```python
from build123d import *

# Parameters (mm, degrees)
ESQUISSE1_R             = 1.5
ESQUISSE1_R_2           = 0.975
BOSS_EXTRU_3_DEPTH      = 2
ESQUISSE2_R             = 1.5
ENL_V_MAT_EXTRU_1_DEPTH = 10


with BuildPart() as part:
    # Esquisse1 → Boss.-Extru.3 (new body)
    with BuildSketch(Plane.XY):
        with BuildLine():
            Line((31.640550531, -4.887241018), (16.450544828, -15.819470843))
            ThreePointArc((16.450544828, -15.819470843), (15.064222472, -16.51996197), (13.529826111, -16.761219719))
            Line((13.529826111, -16.761219719), (-13.529826111, -16.761219719))
            ThreePointArc((-13.529826111, -16.761219719), (-15.064222472, -16.51996197), (-16.450544828, -15.819470843))
            Line((-16.450544828, -15.819470843), (-31.640550531, -4.887241018))
            ThreePointArc((-31.640550531, -4.887241018), (-33.169752802, -3.108946738), (-33.719831815, -0.828989895))
            Line((-33.719831815, -0.828989895), (-33.719831815, 0.549989061))
            ThreePointArc((-33.719831815, 0.549989061), (-33.448369589, 2.175083064), (-32.663459607, 3.623716413))
            Line((-32.663459607, 3.623716413), (-30.727499402, 6.107575779))
            ThreePointArc((-30.727499402, 6.107575779), (-30.464326323, 6.418261685), (-30.17674656, 6.706504084))
            Line((-30.17674656, 6.706504084), (-24.719522272, 11.748000297))
            ThreePointArc((-24.719522272, 11.748000297), (-18.785145606, 15.463312907), (-11.905042981, 16.761219719))
            Line((-11.905042981, 16.761219719), (11.905042981, 16.761219719))
            ThreePointArc((11.905042981, 16.761219719), (18.785145606, 15.463312907), (24.719522272, 11.748000297))
            Line((24.719522272, 11.748000297), (30.17674656, 6.706504084))
            ThreePointArc((30.17674656, 6.706504084), (30.464326323, 6.418261685), (30.727499402, 6.107575779))
            Line((30.727499402, 6.107575779), (32.663459607, 3.623716413))
            ThreePointArc((32.663459607, 3.623716413), (33.448369589, 2.175083064), (33.719831815, 0.549989061))
            Line((33.719831815, 0.549989061), (33.719831815, -0.828989895))
            ThreePointArc((33.719831815, -0.828989895), (33.169752802, -3.108946738), (31.640550531, -4.887241018))
        make_face()
        with Locations((-30.225692015, 2.268354752)):
            Circle(ESQUISSE1_R, mode=Mode.SUBTRACT)
        with Locations((-8.782063878, 13.78106332)):
            Circle(ESQUISSE1_R_2, mode=Mode.SUBTRACT)
        with Locations((-8.782063878, -13.88893668)):
            Circle(ESQUISSE1_R_2, mode=Mode.SUBTRACT)
        with Locations((8.782063878, -13.88893668)):
            Circle(ESQUISSE1_R_2, mode=Mode.SUBTRACT)
        with Locations((8.782063878, 13.78106332)):
            Circle(ESQUISSE1_R_2, mode=Mode.SUBTRACT)
        with Locations((30.225692015, 2.268354752)):
            Circle(ESQUISSE1_R, mode=Mode.SUBTRACT)
        with BuildLine():
            Line((-2.5, 11.487169319), (-2.5, -11.576554556))
            add(Edge.make_bspline(
                [(-2.5, -11.576554556), (-2.473208566, -11.739357127), (-2.553615023, -12.100978181), (-2.87033079, -12.292815757), (-3.033099085, -12.319601551)],
                knots=[0, 0, 0, 0, 0.785398163, 1.570796327, 1.570796327, 1.570796327, 1.570796327], degree=3))
            Line((-3.033099085, -12.319601551), (-14.597943906, -12.285266489))
            add(Edge.make_bspline(
                [(-14.597943906, -12.285266489), (-14.777700694, -12.284097516), (-15.151218557, -12.131430398), (-15.299227824, -11.755845667), (-15.298058605, -11.576051026)],
                knots=[1.570796327, 1.570796327, 1.570796327, 1.570796327, 2.35619449, 3.141592654, 3.141592654, 3.141592654, 3.141592654], degree=3))
            Line((-15.298058605, -11.576051026), (-15.298037902, 11.261063321))
            add(Edge.make_bspline(
                [(-15.298037902, 11.261063321), (-15.29803156, 11.4396883), (-15.148551709, 11.811852348), (-14.776487869, 11.961093545), (-14.597900496, 11.961087204)],
                knots=[0, 0, 0, 0, 0.785398163, 1.570796327, 1.570796327, 1.570796327, 1.570796327], degree=3))
            Line((-14.597900496, 11.961087204), (-11.128260179, 11.961087204))
            Line((-11.128260179, 11.961087204), (-3.087360016, 11.987859762))
            add(Edge.make_bspline(
                [(-3.087360016, 11.987859762), (-2.948581163, 11.998907943), (-2.650223858, 11.905940648), (-2.511050508, 11.625977396), (-2.5, 11.487169319)],
                knots=[1.570796327, 1.570796327, 1.570796327, 1.570796327, 2.35619449, 3.141592654, 3.141592654, 3.141592654, 3.141592654], degree=3))
        make_face(mode=Mode.SUBTRACT)
        with BuildLine():
            Line((3.033099085, -12.319601551), (14.597943906, -12.285266489))
            add(Edge.make_bspline(
                [(14.597943906, -12.285266489), (14.777700694, -12.284097516), (15.151218557, -12.131430398), (15.299227824, -11.755845667), (15.298058605, -11.576051026)],
                knots=[1.570796327, 1.570796327, 1.570796327, 1.570796327, 2.35619449, 3.141592654, 3.141592654, 3.141592654, 3.141592654], degree=3))
            Line((15.298058605, -11.576051026), (15.298037902, 11.261063321))
            add(Edge.make_bspline(
                [(15.298037902, 11.261063321), (15.29803156, 11.4396883), (15.148551709, 11.811852348), (14.776487869, 11.961093545), (14.597900496, 11.961087204)],
                knots=[0, 0, 0, 0, 0.785398163, 1.570796327, 1.570796327, 1.570796327, 1.570796327], degree=3))
            Line((14.597900496, 11.961087204), (11.128260179, 11.961087204))
            Line((11.128260179, 11.961087204), (3.087360016, 11.987859762))
            add(Edge.make_bspline(
                [(3.087360016, 11.987859762), (2.948581163, 11.998907943), (2.650223858, 11.905940648), (2.511050508, 11.625977396), (2.5, 11.487169319)],
                knots=[1.570796327, 1.570796327, 1.570796327, 1.570796327, 2.35619449, 3.141592654, 3.141592654, 3.141592654, 3.141592654], degree=3))
            Line((2.5, 11.487169319), (2.5, -11.576554556))
            add(Edge.make_bspline(
                [(2.5, -11.576554556), (2.473208566, -11.739357127), (2.553615023, -12.100978181), (2.87033079, -12.292815757), (3.033099085, -12.319601551)],
                knots=[0, 0, 0, 0, 0.785398163, 1.570796327, 1.570796327, 1.570796327, 1.570796327], degree=3))
        make_face(mode=Mode.SUBTRACT)
    extrude(amount=BOSS_EXTRU_3_DEPTH)

    # Esquisse2 → Enlèv. mat.-Extru.1 (cut)
    with BuildSketch(Plane.XY.offset(2)):
        with Locations((29.955535999, 19.762236701)):
            Circle(ESQUISSE2_R)
        with Locations((-60.239561974, 19.762236701)):
            Circle(ESQUISSE2_R)
    extrude(amount=-ENL_V_MAT_EXTRU_1_DEPTH, mode=Mode.SUBTRACT)


solid = part.part
```
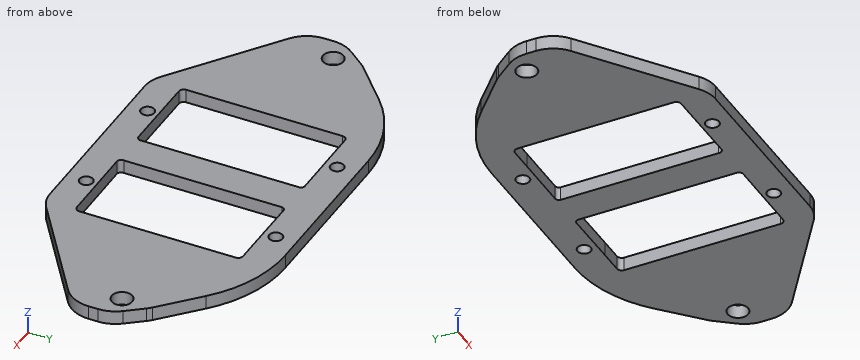
Here's how the part is built. I have some questions about the finished solid (model axes, mm). Coordinates: 2 decimals unless noted, no trailing zeros. Order: outer loops, then holes, each group sorted by start corner. A loop starts at its lowest first (then second) coordinate and runs counter-clockwise, first axis right, second up.
Item 1: I'm going to push flat-ended pins straight in: pin 1 Ø1 at (y, z) = (2.5, 1) entering from -X; pin 2 Ø1 at (y, z) = (-1.5, 1.5) entering from +X; pin 3 Ø1 at (y, z) = (-3, 0.5) entering from +X. Where does each tip first touch, or does it pass through?
Response values:
pin 1: stops at x = -33.5
pin 2: stops at x = 33.72
pin 3: stops at x = 33.43
Item 2: If we section it at D-D, the plane z = 0.65: Give the number of separate pieces and of enclosed holes in the cut face, then the cut area to 3 significant figures.
Response values:
separate pieces: 1
enclosed holes: 8
area: 1,150 mm2
Item 3: I need wall thicknesses on probe 1 along Y at (x, z) = (3, 1.3); probe 2 along X at (y, z) = (9, 1.3); probe 3 along X at (y, z) = (-12, 1.3). Which ranges of each line are inside material? Lowest first, please.
Response values:
probe 1: y = -16.76 to -12.31, 11.99 to 16.76
probe 2: x = -27.69 to -15.3, -2.5 to 2.5, 15.3 to 27.69
probe 3: x = -21.76 to -15.16, -2.58 to 2.58, 15.16 to 21.76
Item 4: If we section it at B-B, the plane x = -6: List the corners of the cut face in (y, z) for me.
Response values:
outline: (-16.76, 0) - (-12.31, 0) - (-12.31, 2) - (-16.76, 2) - close; (11.98, 0) - (16.76, 0) - (16.76, 2) - (11.98, 2) - close
Item 5: If we section it at C-C, the plane y = -3: List the corners of the cut face in (x, z) for me.
Response values:
outline: (-33.22, 0) - (-15.3, 0) - (-15.3, 2) - (-33.22, 2) - close; (-2.5, 0) - (2.5, 0) - (2.5, 2) - (-2.5, 2) - close; (15.3, 0) - (33.22, 0) - (33.22, 2) - (15.3, 2) - close
Item 6: If we section it at A-A, the plane y = 4.5: List the corners of the cut face in (x, z) for me.
Response values:
outline: (-31.98, 0) - (-15.3, 0) - (-15.3, 2) - (-31.98, 2) - close; (-2.5, 0) - (2.5, 0) - (2.5, 2) - (-2.5, 2) - close; (15.3, 0) - (31.98, 0) - (31.98, 2) - (15.3, 2) - close
